Input: part model. Units: mm. Frame: model coordinates. A direction names the side the tool comes from. Coordinates: 2 decimals unless noted, no trailing zeros. Loops run counter-clockwise (first coordinate to the right, second up) from the corner with the lowest first, then second, coordinate; pieces in that order, holes last.
```python
from build123d import *

# Parameters (mm, degrees)
SKETCH1_W           = 90
SKETCH1_H           = 60
BOSS_EXTRUDE1_DEPTH = 50
SHELL1_T            = -3
CUT_EXTRUDE1_DEPTH  = 90
BOSS_EXTRUDE2_DEPTH = 90


with BuildPart() as part:
    # Sketch1 → Boss-Extrude1 (new body)
    with BuildSketch(Plane(origin=(0, 0, 0), x_dir=(1, 0, 0), z_dir=(0, 1, 0))):
        Rectangle(SKETCH1_W, SKETCH1_H)
    extrude(amount=BOSS_EXTRUDE1_DEPTH)

    # Shell1
    shell1_openings = [part.faces().sort_by_distance(p)[0] for p in [
        (0, 50, 0),
    ]]
    offset(amount=SHELL1_T, openings=shell1_openings, kind=Kind.INTERSECTION)

    # Sketch2 → Cut-Extrude1 (cut)
    with BuildSketch(Plane.ZY.offset(45)):
        with BuildLine():
            Line((-30, 25), (-12.94347358, 25))
            ThreePointArc((-12.94347358, 25), (-3.791055639, 28.791055639), (0, 37.94347358))
            Line((0, 37.94347358), (0, 50))
            Line((0, 50), (-30, 50))
            Line((-30, 50), (-30, 25))
        make_face()
    extrude(amount=-CUT_EXTRUDE1_DEPTH, mode=Mode.SUBTRACT)

    # Sketch3 → Boss-Extrude2 (add)
    with BuildSketch(Plane.ZY.offset(45)):
        Polygon((30, 50), (40, 50), (40, 47.197660371), (30, 42.867982808), (30, 44.997500312), (37, 48.028274606), (30, 48.028274606), align=None)
    extrude(amount=-BOSS_EXTRUDE2_DEPTH)


solid = part.part
```
Item 1: Reachability of faces 4 (the face through (-42, 21, 6)), 5 (the face through (-1, 12, -30)) from +Z, -Z, +X, -X, +Y, -Y: full face, straight path, thin tool, end or side. Return the list, or none.
Result:
face 4: +Y
face 5: -Z, +X, -X, +Y, -Y
Item 2: Line query: L1, parallel to Z at x = 0, y = 12; L2, parallel to X at y = 21, z = 15; L3, parallel to Z at x = -30, y = 27.5. Output: solid intervals per line, ascending.
Result:
L1: z = -30 to -27, 27 to 30
L2: x = -45 to -42, 42 to 45
L3: z = 27 to 30
Item 3: Mould query, pull axis Y, two halves, no side actions, for faces 1 (the face through (-1, 46, 30)), 2 (the face through (0, 50, 30)), 3 (the face through (43, 44, 0)). Classes: +Y half, -Y half, draft (parallel to the pull), parting line (faces both ways), or undercut.
Result:
face 1: undercut
face 2: +Y half
face 3: draft
Item 4: Contact query for flat-ended pins moving along their axis: P1, Ø8, axis at x = -3.5, y = 39.5, coming from the -Z side; P2, Ø5, axis at y = 29, z = 33, coming from the -X side; P3, Ø19, axis at x = -9, z = -21.5, coming from the +Y side; P4, Ø11, axis at x = 12.5, y = 14.5, coming from the +Z side. Output: stop coordinate, or through.
Result:
P1: stops at z = 27
P2: passes through
P3: stops at y = 25
P4: stops at z = 30
Item 5: Section query B-B (x = 5). Output: boundary loops of the cut face in (y, z), then the cut area to 3 significant figures.
Result:
outline: (0, -30) - (25, -30) - (25, -27) - (3, -27) - (3, 27) - (50, 27) - (50, 40) - (47.2, 40) - (42.87, 30) - (0, 30) - close; hole (45, 30) - (48.03, 30) - (48.03, 37) - close
area: 426 mm2
Item 6: Section query A-A (y = 18). Output: boundary loops of the cut face in (x, z), then the cut area to 3 significant figures.
Result:
outline: (-45, -30) - (45, -30) - (45, 30) - (-45, 30) - close; hole (-42, -27) - (42, -27) - (42, 27) - (-42, 27) - close
area: 864 mm2
Item 7: Section query D-D (y = 46). Output: boundary loops of the cut face in (x, z).
Result:
outline: (-45, 0) - (-42, 0) - (-42, 27) - (42, 27) - (42, 0) - (45, 0) - (45, 30) - (-45, 30) - close; (-45, 32.32) - (45, 32.32) - (45, 37.23) - (-45, 37.23) - close
Item 8: Section query C-C (z = -25). Output: boundary loops of the cut face in (x, y).
Result:
outline: (-45, 0) - (45, 0) - (45, 25) - (42, 25) - (42, 3) - (-42, 3) - (-42, 25) - (-45, 25) - close
